from build123d import *

# Parameters (mm, degrees)
SKETCH1_R           = 1.8
BOSS_EXTRUDE2_DEPTH = 5


with BuildPart() as part:
    # Sketch1 → Boss-Extrude2 (new body)
    with BuildSketch(Plane.XY):
        with BuildLine():
            Line((4, 0), (50, 0))
            ThreePointArc((50, 0), (56.064971157, -13.642135624), (70, -19))
            Line((70, -19), (90, -19))
            Line((90, -19), (90, -9))
            Line((90, -9), (69.8490214, -9))
            ThreePointArc((69.8490214, -9), (62.990773359, -6.428332012), (59.996714309, 0.256326008))
            Line((59.996714309, 0.256326008), (59.996714309, 11.743673992))
            ThreePointArc((59.996714309, 11.743673992), (62.990773359, 18.428332012), (69.8490214, 21))
            Line((69.8490214, 21), (90, 21))
            Line((90, 21), (90, 31))
            Line((90, 31), (70, 31))
            ThreePointArc((70, 31), (56.064971157, 25.642135624), (50, 12))
            Line((50, 12), (4, 12))
            Line((4, 12), (0, 8))
            Line((0, 8), (0, 4))
            Line((0, 4), (4, 0))
        make_face()
        with Locations((6, 6)):
            Circle(SKETCH1_R, mode=Mode.SUBTRACT)
    extrude(amount=BOSS_EXTRUDE2_DEPTH)


solid = part.part
Source: CAD feature listing. Evaluate the final solid. Frame: model axes, mm. A direction names the side the tool comes from. Round coordinates to 2 decimals unless told otherwise and drop trailing zeros. Loops run counter-clockwise (first coordinate to the right, second up) from the corner with the lowest first, then second, coordinate; pieces in that order, holes last. Notation, with made-up numbers: (51, 7) - (104, 7) arc R13 cw to (104, 31) - close; hole circle Ø1 at (43.5, -30). An arc over 180 degrees is marked (long way). Write item = value, one per line. Start each with the question number.
Item 1: Section query D-D on x = 21.5. Output: boundary loops of the cut face in (y, z), plus the area to 3 significant figures.
Item 2: Section query A-A on y = 6. Output: boundary loops of the cut face in (x, z), plus the area to 3 significant figures.
Item 3: First-contact query: pin 1 Ø2.5 at (x, z) = (79.5, 2) entering from +Y; pin 2 Ø1.5 at (x, z) = (16.5, 4) entering from -Y; pin 3 Ø2.5 at (x, z) = (78, 3) entering from -Y. Flat tips, straight axial feed; report the tip coordinate or a pass-through.
Item 4: Reachability of faces 1 (the face through (27, 0, 2)), 2 (the face through (54, 6, 0)), 3 (the face through (59.997, 6, 2)) from +Z, -Z, +X, -X, +Y, -Y: full face, straight path, thin tool, end or side. Return the list, or none.
Item 5: Material intervals for line 1 (Y direction, x = 6, z = 3.9); line 2 (Y direction, x = 81.5, z = 2.75); line 3 (Y direction, x = 28.5, z = 3.05), sorted ascending.
Item 6: Mould query, pull axis Y, two halves, no side actions, for faces 4 (the face through (62.914, 18.356, 2.465)), 5 (the face through (27, 12, 2)), 6 (the face through (90, 26, 2)). Classes: released by +Y, released by -Y, zero draft, split by the parting line, or undercut.
Item 7: Section query C-C on z = 4.25. Output: boundary loops of the cut face in (x, y).
Item 8: Section query B-B on x = 6. Output: boundary loops of the cut face in (y, z).
Results list:
q1.outline = (0, 0) - (12, 0) - (12, 5) - (0, 5) - close
q1.area = 60.0 mm²
q2.outline = (0, 0) - (4.2, 0) - (4.2, 5) - (0, 5) - close; (7.8, 0) - (60, 0) - (60, 5) - (7.8, 5) - close
q2.area = 282 mm²
q3.pin_1 = 31
q3.pin_2 = 0
q3.pin_3 = -19
q4.face_1 = +Z, -Z, -X, -Y
q4.face_2 = -Z, +X, -X, +Y, -Y
q4.face_3 = +Z, -Z, +X
q5.line_1 = 0 to 4.2, 7.8 to 12
q5.line_2 = -19 to -9, 21 to 31
q5.line_3 = 0 to 12
q6.face_4 = undercut
q6.face_5 = released by +Y
q6.face_6 = zero draft
q7.outline = (0, 4) - (4, 0) - (50, 0) arc R19.51 ccw to (70, -19) - (90, -19) - (90, -9) - (69.85, -9) arc R9.51 cw to (60, 0.26) - (60, 11.74) arc R9.51 cw to (69.85, 21) - (90, 21) - (90, 31) - (70, 31) arc R19.51 ccw to (50, 12) - (4, 12) - (0, 8) - close; hole circle Ø3.6 at (6, 6)
q8.outline = (0, 0) - (4.2, 0) - (4.2, 5) - (0, 5) - close; (7.8, 0) - (12, 0) - (12, 5) - (7.8, 5) - close
